Autodesk Fusion 360 part; units mm, degrees
sketch "Sketch1" plane through (0, 0, 0) normal (0, 0, 1) x (1, 0, 0)
  circle A0 centre (0, 0) radius 2.95
  dimension "d1" = 5.9
extrude "Extrude1" add sketch "Sketch1" along normal blind 12
sketch "Sketch2" plane through (0, 0, 12) normal (0, 0, 1) x (-1, 0, 0)
  circle A0 centre (0, 0) radius 2.95
  circle A1 centre (0, 0) radius 4.084
extrude "Extrude2" add sketch "Sketch2" along normal blind 3 contours A0 | A1
sketch "Sketch3" plane through (0, 0, 15) normal (0, 0, 1) x (-1, 0, 0)
  circle A0 centre (0, 0) radius 4.084
  circle A1 centre (0, 0) radius 1.75
  dimension "d6" = 3.5
extrude "Extrude3" cut sketch "Sketch3" against normal blind 4 contours A1
fillet "Fillet1" radius 1 1 edges at (-2.7504, -1.0668, 0)
fillet "Fillet2" radius 1 1 edges at (1.6316, -0.6328, 15)
Read the model definition and answer for the solid it produces. Units are mm, in the model's axes. A direction names the side the tool comes from. Give positions to 0.01 mm unless a question says otherwise; leave off trailing zeros. Write each loop counter-clockwise with the first axis right and the second up, starting at its lowest first coordinate (ties: lowest second). Pieces come first, ordered by that corner, then holes. Notation, with made-up numbers: (1, -20.75) - (21, -20.75) arc R15 ccw to (21, -0.75) - close; hole circle Ø4 at (87.25, 34). An arc over 180 degrees is marked (long way). Write item = value, one per line. Start each with the question number.
Item 1: A tool of negligible diameter and unlimited length cuts with its end or side. For faces 4 (the cylindrical face through (-2.947, -0.13, 6.423)), 5 (the flat face through (0, 0, 0)), 6 (the flat face through (0, 0, 11)), from which of +Z, -Z, +X, -X, +Y, -Y can it reach the whole face along a straight path? Write none if from no direction.
Item 2: Find section C-C (z = 10). Give the vertices of the cut face in (x, y), then the cut area to 3 significant figures.
Item 3: The mould has two halves that part along Y. Classify faces 1 (the cylindrical face through (-3.895, 1.227, 13.479)), 2 (the cylindrical face through (-1.617, 0.67, 12.521)), 3 (the flat face through (-1, 3, 12)): +Y half, -Y half, draft (parallel to the pull), parting line (faces both ways), or undercut.
Item 4: Find section A-A (y = 0). Give the vertices of the cut face in (x, z), then the cut area to 3 significant figures.
Item 5: Find section D-D (z = 13.75). Give the vertices of the cut face in (x, y), then the cut area to 3 significant figures.
Item 6: Find the intervals of material crossed by probe 1 along X at (y, z) = (0, 13.1); probe 2 along Z at (x, y) = (2.75, -2.75), in increasing order. Write a range as [from, to].
Item 7: Each of these flat-tipped pins is pushed along its axis until it touches: P1, Ø4, axis at y = 3, z = 7, coming from the +X side; P2, Ø1, axis at y = -2.5, z = 8.5, coming from the -X side; P3, Ø4.5, axis at x = 0, y = 0, coming from the +Z side. Where does it stop, or does it pass through?
Response:
q1.face_4 = -Z
q1.face_5 = -Z, +X, -X, +Y, -Y
q1.face_6 = +Z
q2.outline = circle Ø5.9 at (0, 0)
q2.area = 27.3 mm²
q3.face_1 = parting line
q3.face_2 = undercut
q3.face_3 = draft
q4.outline = (-4.08, 12) - (-2.95, 12) - (-2.95, 1) arc R1 ccw to (-1.95, 0) - (1.95, 0) arc R1 ccw to (2.95, 1) - (2.95, 12) - (4.08, 12) - (4.08, 15) - (2.75, 15) arc R1 ccw to (1.75, 14) - (1.75, 11) - (-1.75, 11) - (-1.75, 14) arc R1 ccw to (-2.75, 15) - (-4.08, 15) - close
q4.area = 80.4 mm²
q5.outline = circle Ø8.17 at (0, 0); hole circle Ø3.5 at (0, 0)
q5.area = 42.8 mm²
q6.probe_1 = [-4.08, -1.75], [1.75, 4.08]
q6.probe_2 = [12, 15]
q7.P1 = 2.78
q7.P2 = -2.17
q7.P3 = 14.87
